The model under review builds one solid part; all positions refer to its coordinate system, in mm. A direction names the side the tool comes from. Coordinates: 2 decimals unless noted, no trailing zeros. Loops run counter-clockwise (first coordinate to the right, second up) from the corner with the lowest first, then second, coordinate; pieces in that order, holes last. Notation, with made-up numbers: M -18.5,1 L 24.5,1 A29 ccw 24.5,24 Z; hole C 42,36.25 d5. An arc over 180 degrees is marked long. Use one line per item in the form item = value.
```python
from build123d import *

# Parameters (mm, degrees)
SKETCH1_R             = 10.35
SKETCH1_R_2           = 4.4
SKETCH1_R_3           = 0.75
BOSS_EXTRUDE1_DEPTH   = 2
CIRPATTERN2_OUTLINE_R = 0.75
CIRPATTERN2_DEPTH     = 2
SKETCH1_2_R           = 4.4
BOSS_EXTRUDE2_DEPTH   = 4.5
SKETCH2_R             = 1.5
CUT_EXTRUDE1_DEPTH    = 4.5
SKETCH3_R             = 2.75
CUT_EXTRUDE2_DEPTH    = 3.5
CUT_EXTRUDE3_DEPTH    = 3.5
CIRPATTERN1_COUNT     = 25


# Read off the part's stored shape, not the designer's step: CirPattern2
with BuildPart() as part:
    # Sketch1 → Boss-Extrude1 (new body)
    with BuildSketch(Plane.XY):
        Circle(SKETCH1_R)
        Circle(SKETCH1_R_2, mode=Mode.SUBTRACT)
        with Locations((0, 7.247764581)):
            Circle(SKETCH1_R_3, mode=Mode.SUBTRACT)
        with Locations((3.5, 7.247764581)):
            Circle(SKETCH1_R_3, mode=Mode.SUBTRACT)
        with Locations((-3.5, 7.247764581)):
            Circle(SKETCH1_R_3, mode=Mode.SUBTRACT)
    extrude(amount=BOSS_EXTRUDE1_DEPTH)

    # CirPattern2 outline → CirPattern2 (cut)
    with BuildSketch(Plane.XY):
        with Locations((7.247764581, 3.5)):
            Circle(CIRPATTERN2_OUTLINE_R)
        with Locations((7.247764581, 0)):
            Circle(CIRPATTERN2_OUTLINE_R)
        with Locations((7.247764581, -3.5)):
            Circle(CIRPATTERN2_OUTLINE_R)
        with Locations((3.5, -7.247764581)):
            Circle(CIRPATTERN2_OUTLINE_R)
        with Locations((0, -7.247764581)):
            Circle(CIRPATTERN2_OUTLINE_R)
        with Locations((-3.5, -7.247764581)):
            Circle(CIRPATTERN2_OUTLINE_R)
        with Locations((-7.247764581, -3.5)):
            Circle(CIRPATTERN2_OUTLINE_R)
        with Locations((-7.247764581, 0)):
            Circle(CIRPATTERN2_OUTLINE_R)
        with Locations((-7.247764581, 3.5)):
            Circle(CIRPATTERN2_OUTLINE_R)
    extrude(amount=CIRPATTERN2_DEPTH, mode=Mode.SUBTRACT)

    # Sketch1<2> → Boss-Extrude2 (add)
    with BuildSketch(Plane.XY):
        Circle(SKETCH1_2_R)
    extrude(amount=BOSS_EXTRUDE2_DEPTH)

    # Sketch2 → Cut-Extrude1 (cut)
    with BuildSketch(Plane(origin=(0, 0, 0), x_dir=(-1, 0, 0), z_dir=(0, 0, -1))):
        Circle(SKETCH2_R)
    extrude(amount=-CUT_EXTRUDE1_DEPTH, mode=Mode.SUBTRACT)

    # Sketch3 → Cut-Extrude2 (cut)
    with BuildSketch(Plane.XY.offset(4.5)):
        Circle(SKETCH3_R)
    extrude(amount=-CUT_EXTRUDE2_DEPTH, mode=Mode.SUBTRACT)

    # Sketch4 → Cut-Extrude3 (cut)
    with BuildSketch(Plane.XY.offset(4.5)):
        with BuildLine():
            Line((-2.976344104, 0.375999701), (-2.728315429, 0.344666392))
            ThreePointArc((-2.728315429, 0.344666392), (-2.70218519, 0.510583192), (-2.665974712, 0.674595311))
            Line((-2.665974712, 0.674595311), (-2.976344104, 0.375999701))
        make_face()
        with BuildLine():
            Line((-2.976344104, 0.375999701), (-2.75, 0))
            ThreePointArc((-2.75, 0), (-2.744573503, 0.172673929), (-2.728315429, 0.344666392))
            Line((-2.728315429, 0.344666392), (-2.976344104, 0.375999701))
        make_face()
    cut_extrude3 = extrude(amount=-CUT_EXTRUDE3_DEPTH, mode=Mode.SUBTRACT)

    # CirPattern1: Cut-Extrude3 ×25 about axis
    cirpattern1_axis = Axis((0, 0, 0), (0, 0, 1))
    for i in range(1, CIRPATTERN1_COUNT):
        add(cut_extrude3.rotate(cirpattern1_axis, i * 360 / CIRPATTERN1_COUNT), mode=Mode.SUBTRACT)


solid = part.part
```
1. Insertion check: P1, Ø1, axis at x = -1, y = 5, coming from the +Z side; P2, Ø0.9, axis at x = 3.5, y = -7.25, coming from the -Z side; P3, Ø1.8, axis at x = -1, y = -1, coming from the +Z side; P4, Ø1.5, axis at y = 3.5, z = 3.5, coming from the +X side. Each pin has a flat end and moves straight along its axis. Give the tip position at first contact, or say it passes through.
Response values:
P1 = 2
P2 = through
P3 = 1
P4 = 3.43
2. Wall thickness on line 1 along Y through (x, z) = (0, 0.55); line 2 along Y through (x, z) = (0, 1.2); line 3 along X through (y, z) = (-7, 1.5): over which ranges is each line inside the solid? List them lowest first. Write a range as from..to.
Response values:
line_1 = -10.35..-8, -6.5..-1.5, 1.5..6.5, 8..10.35
line_2 = -10.35..-8, -6.5..-2.86, 2.86..6.5, 8..10.35
line_3 = -7.62..-4.21, -2.79..-0.71, 0.71..2.79, 4.21..7.62
3. Add section D-D (y = 6). State the section outline as (x, z) points.
Response values:
outline = M -8.43,0 L 8.43,0 L 8.43,2 L -8.43,2 Z
4. Machinability: for faces 4 (the face through (-3.6, 7.99, 0.99)), 5 (the face through (1.3, 1.4, 1)), which of the approach directions +Z, -Z, +X, -X, +Y, -Y give a long, thin tool a straight path to every point of the face, cutting with its end or side? Answer none if there is none.
Response values:
face_4 = +Z, -Z
face_5 = +Z
5. Add section C-C (y = 8.25). State the section outline as (x, z) points.
Response values:
outline = M -6.25,0 L 6.25,0 L 6.25,2 L -6.25,2 Z
6. Add section B-B (z = 0.7). Count the separate pieces of the cut face and the enclosed holes in it, then the cut area to 3 significant figures.
Response values:
separate_pieces = 1
enclosed_holes = 13
area = 308 mm^2
7. The part is to be moulded in two halves that separate along X. For faces 1 (the face through (1, -3, 4.5)), 2 (the face through (4.197, 1.322, 3.232)), 3 (the face through (-4.1, -7.7, 1)), say which applies: pulls with the +X half, pulls with the -X half, needs draft (parallel to the pull), parting line crosses it, or undercut.
Response values:
face_1 = needs draft
face_2 = parting line crosses it
face_3 = undercut
8. Add section A-A (x = 3.5). State the section outline as (y, z) points, then the cut area to 3 significant figures.
Response values:
outline = M -9.74,0 L -8,0 L -8,2 L -9.74,2 Z; M -6.5,0 L 6.5,0 L 6.5,2 L 2.67,2 L 2.67,4.5 L -2.67,4.5 L -2.67,2 L -6.5,2 Z; M 8,0 L 9.74,0 L 9.74,2 L 8,2 Z
area = 46.3 mm^2
